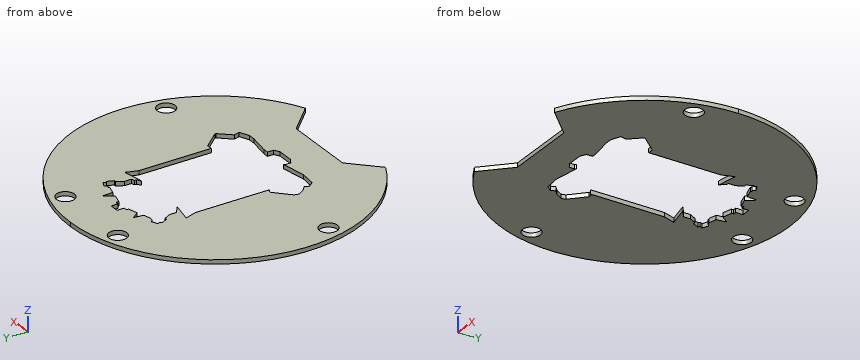
from build123d import *

# Parameters (mm, degrees)
F0_R     = 6.5
F1_DEPTH = 3


with BuildPart() as f1:
    # F0 (on Top) → F1 (new body)
    with BuildSketch(Plane.XY):
        with BuildLine():
            Line((0, 72.78838), (0, 105))
            ThreePointArc((0, 105), (-102.419357, 23.136018), (-45.134783, -94.804279))
            Line((-45.134783, -94.804279), (-26.122815, -75.792312))
            Line((-26.122815, -75.792312), (0, -75.792312))
            Line((0, -75.792312), (0, -64.716025))
            Line((0, -64.716025), (0, -51.507495))
            Line((0, -51.507495), (-4.902991, -51.507495))
            Line((-4.902991, -51.507495), (-8.982703, -49.268302))
            Line((-8.982703, -49.268302), (-8.982703, -45.383053))
            Line((-8.982703, -45.383053), (-8.322856, -44.464201))
            Line((-8.322856, -44.464201), (-26.155021, -47.517654))
            Line((-26.155021, -47.517654), (-37.188161, -46.499837))
            Line((-37.188161, -46.499837), (-40.241614, -42.713556))
            Line((-40.241614, -42.713556), (-38.775958, -39.660104))
            Line((-38.775958, -39.660104), (-42.032976, -36.932353))
            Line((-42.032976, -36.932353), (-45.260154, -31.819914))
            Line((-45.260154, -31.819914), (-44.569235, -28.768361))
            Line((-44.569235, -28.768361), (-34.090322, -18.546099))
            Line((-34.090322, -18.546099), (-32.151641, -18.546099))
            Line((-32.151641, -18.546099), (-30.825328, -19.498551))
            Line((-30.825328, -19.498551), (-30.825328, 34.089174))
            Line((-30.825328, 34.089174), (-33.692077, 42.6598))
            Line((-33.692077, 42.6598), (-18.384103, 39.402783))
            Line((-18.384103, 39.402783), (-24.450295, 43.759041))
            Line((-24.450295, 43.759041), (-24.450295, 48.807416))
            Line((-24.450295, 48.807416), (-26.969282, 53.710941))
            Line((-26.969282, 53.710941), (-28.595109, 53.710941))
            Line((-28.595109, 53.710941), (-30.825328, 58.393094))
            Line((-30.825328, 58.393094), (-29.480881, 59.033486))
            Line((-29.480881, 59.033486), (-30.429862, 61.025791))
            Line((-30.429862, 61.025791), (-26.284034, 63.000545))
            Line((-26.284034, 63.000545), (-24.078682, 61.416837))
            Line((-24.078682, 61.416837), (-22.965606, 61.416837))
            Line((-22.965606, 61.416837), (-22.421065, 61.025791))
            Line((-22.421065, 61.025791), (-16.709682, 62.528782))
            Line((-16.709682, 62.528782), (-15.732577, 69.490649))
            Line((-15.732577, 69.490649), (-11.864871, 64.198002))
            Line((-11.864871, 64.198002), (-4.902991, 66.03007))
            Line((-4.902991, 66.03007), (-4.902991, 67.536443))
            Line((-4.902991, 67.536443), (-2.50095, 67.536443))
            Line((-2.50095, 67.536443), (-2.50095, 72.78838))
            Line((-2.50095, 72.78838), (0, 72.78838))
        make_face()
        with Locations((-91.313913, -23.465414)):
            Circle(F0_R, mode=Mode.SUBTRACT)
        with Locations((-29.72243, 89.777015)):
            Circle(F0_R, mode=Mode.SUBTRACT)
        with BuildLine():
            ThreePointArc((45.134783, -94.804279), (88.781057, -56.061787), (105, 0))
            ThreePointArc((105, 0), (74.246212, 74.246212), (0, 105))
            Line((0, 105), (0, 72.78838))
            Line((0, 72.78838), (4.135221, 72.78838))
            Line((4.135221, 72.78838), (4.135221, 67.821436))
            Line((4.135221, 67.821436), (6.415132, 67.821436))
            Line((6.415132, 67.821436), (6.415132, 65.785795))
            Line((6.415132, 65.785795), (13.244115, 63.752693))
            Line((13.244115, 63.752693), (17.773977, 70.060633))
            Line((17.773977, 70.060633), (18.221818, 62.528782))
            Line((18.221818, 62.528782), (24.691317, 60.566589))
            Line((24.691317, 60.566589), (25.253858, 61.34994))
            Line((25.253858, 61.34994), (26.344692, 60.566589))
            Line((26.344692, 60.566589), (27.870728, 62.691629))
            Line((27.870728, 62.691629), (32.310771, 60.566589))
            Line((32.310771, 60.566589), (31.013132, 58.759595))
            Line((31.013132, 58.759595), (32.186273, 58.294658))
            Line((32.186273, 58.294658), (30.294107, 53.5203))
            Line((30.294107, 53.5203), (28.80712, 53.856976))
            Line((28.80712, 53.856976), (26.201509, 48.849314))
            Line((26.201509, 48.849314), (26.201509, 43.759041))
            Line((26.201509, 43.759041), (23.840172, 43.149535))
            Line((23.840172, 43.149535), (23.840172, 41.765302))
            Line((23.840172, 41.765302), (21.07171, 39.811093))
            Line((21.07171, 39.811093), (35.768993, 42.375993))
            Line((35.768993, 42.375993), (32.959819, 34.089174))
            Line((32.959819, 34.089174), (32.959819, -17.675241))
            Line((32.959819, -17.675241), (32.959819, -18.546099))
            Line((32.959819, -18.546099), (36.990378, -18.546099))
            Line((36.990378, -18.546099), (47.331408, -30.377604))
            Line((47.331408, -30.377604), (47.331408, -31.232571))
            Line((47.331408, -31.232571), (39.921697, -39.741524))
            Line((39.921697, -39.741524), (41.061651, -43.975644))
            Line((41.061651, -43.975644), (34.09978, -47.06981))
            Line((34.09978, -47.06981), (29.336393, -47.06981))
            Line((29.336393, -47.06981), (14.557681, -44.789899))
            Line((14.557681, -44.789899), (10.404986, -44.789899))
            Line((10.404986, -44.789899), (10.404986, -49.268302))
            Line((10.404986, -49.268302), (6.496566, -51.507495))
            Line((6.496566, -51.507495), (0, -51.507495))
            Line((0, -51.507495), (0, -64.716025))
            Line((0, -64.716025), (0, -75.792312))
            Line((0, -75.792312), (26.122815, -75.792312))
            Line((26.122815, -75.792312), (45.134783, -94.804279))
        make_face()
        with Locations((91.313914, -23.465414)):
            Circle(F0_R, mode=Mode.SUBTRACT)
        with Locations((29.297218, 89.777015)):
            Circle(F0_R, mode=Mode.SUBTRACT)
    extrude(amount=F1_DEPTH)


solid = f1.part
Part model, mm, in its own coordinate system. Coordinates: 2 decimals unless noted, no trailing zeros. Loops run counter-clockwise (first coordinate to the right, second up) from the corner with the lowest first, then second, coordinate; pieces in that order, holes last. Notation, with made-up numbers: (38.5, 50) -> (92.5, 50) arc R16 cw to (92.5, 59) -> close; hole circle Ø1 at (46.5, 21). An arc over 180 degrees is marked (long way). Use a Markdown table: item, result. Add a question column.
Item 1: Band-saw the part on C-C on y = -82.5. Write the cut outline in (x, z).
Item 2: Band-saw the part on D-D on x = 75.5. Write the cut outline in (y, z).
Item 3: Probe probe 1 along Y at (x, z) = (29, 2.7); probe 2 along X at (y, z) = (89, 2.1); probe 3 along Y at (x, z) = (21.5, 2.8). List the from-to ranges inside material, lowest first.
Item 4: Flat gauge pins, fed straight in: P1, Ø2, axis at x = 44, y = -71.5, coming from the -Z side; P2, Ø0.5, axis at x = -28, z = 2, coming from the +Y side; P3, Ø1, axis at x = -66.5, z = 2, coming from the -Y side; P4, Ø0.7, axis at y = -30.5, z = 2, coming from the -X side. Where does each tip first touch, or does it go through?
Item 5: Band-saw the part on B-B on z = 1.9. Give the number of separate pieces and of enclosed holes in the cut face, plus the area to 3 significant figures.
Item 6: Band-saw the part on A-A on y = -4. Write the cut outline in (x, z), plus the area to 3 significant figures.
Geometry says:
| question | item | result |
|---|---|---|
| 1 | outline | (-64.95, 0) -> (-32.83, 0) -> (-32.83, 3) -> (-64.95, 3) -> close; (32.83, 0) -> (64.95, 0) -> (64.95, 3) -> (32.83, 3) -> close |
| 2 | outline | (-72.97, 0) -> (72.97, 0) -> (72.97, 3) -> (-72.97, 3) -> close |
| 3 | probe 1 | -78.67 to -47.02, 41.19 to 53.81, 62.15 to 83.28, 96.27 to 100.92 |
| 3 | probe 2 | -55.71 to -36.18, -23.27 to 22.84, 35.75 to 55.71 |
| 3 | probe 3 | -75.79 to -45.86, 39.89 to 40.11, 61.53 to 102.78 |
| 4 | P1 | z = 0 |
| 4 | P2 | y = 101.27 |
| 4 | P3 | y = -81.66 |
| 4 | P4 | x = -100.58 |
| 5 | separate pieces | 1 |
| 5 | enclosed holes | 5 |
| 5 | area | 24,600 mm² |
| 6 | outline | (-104.92, 0) -> (-30.83, 0) -> (-30.83, 3) -> (-104.92, 3) -> close; (32.96, 0) -> (104.92, 0) -> (104.92, 3) -> (32.96, 3) -> close |
| 6 | area | 438 mm² |
